Design review of the part shown in the three views and the two pictorial views. Dimensions are in mm from the part's minimum x, y and z. A direction names the side the tool comes from. Coordinates: 2 decimals unless noted, no trailing zeros. Loops run counter-clockwise (first coordinate to the right, second up) from the corner with the lowest first, then second, coordinate; pieces in that order, holes last. Notation, with made-up numbers: M 19.25,82 L 61.25,82 A34 cw 61.25,121 Z; hole C 30,76 d2. An arc over 180 degrees is marked long. Put each result on its own line as item: value. Start each with the question number.
(1) Take a section at D-D, the plane z = 43.5. Give the boundary of the cut face in (x, y), then the cut area to 3 significant figures.
(2) Take a section at A-A, the plane y = 6.35. Give the boundary of the cut face in (x, z) (3 decimals), then the cut area to 3 significant figures.
(3) Clearance check with flat-ended pins moving along their axes: pin 1 (1 mm diameter, centred on x = 5, y = 2, fed in from -Z); pin 2 (1.5 mm diameter, centred on x = 5, z = 12, fed in from -Y); pin 3 (4 mm diameter, centred on x = 5.5, y = 9.5, fed in from -Z); pin 4 (1 mm diameter, centred on y = 3, z = 27.5, fed in from +X). State where each tip first meets the part, or that it passes through.
(4) For probe 1 along Z at (x, y) = (7, 1.5); probe 2 along Y at (x, z) = (6.5, 34.5), list the stretches that pass through material, from the lowest coordinate up. Write a range as [from, to].
(5) For the marked faces 1, 2 and 3, list the 3-axis set-ups (+Z, -Z, +X, -X, +Y, -Y) from which the entire face can be reached by the end or side of a thin tool; tool diameter is ignored.
(6) Take a section at C-C, the plane z = 10.5. Give the boundary of the cut face in (x, y) (3 decimals), then the cut area to 3 significant figures.
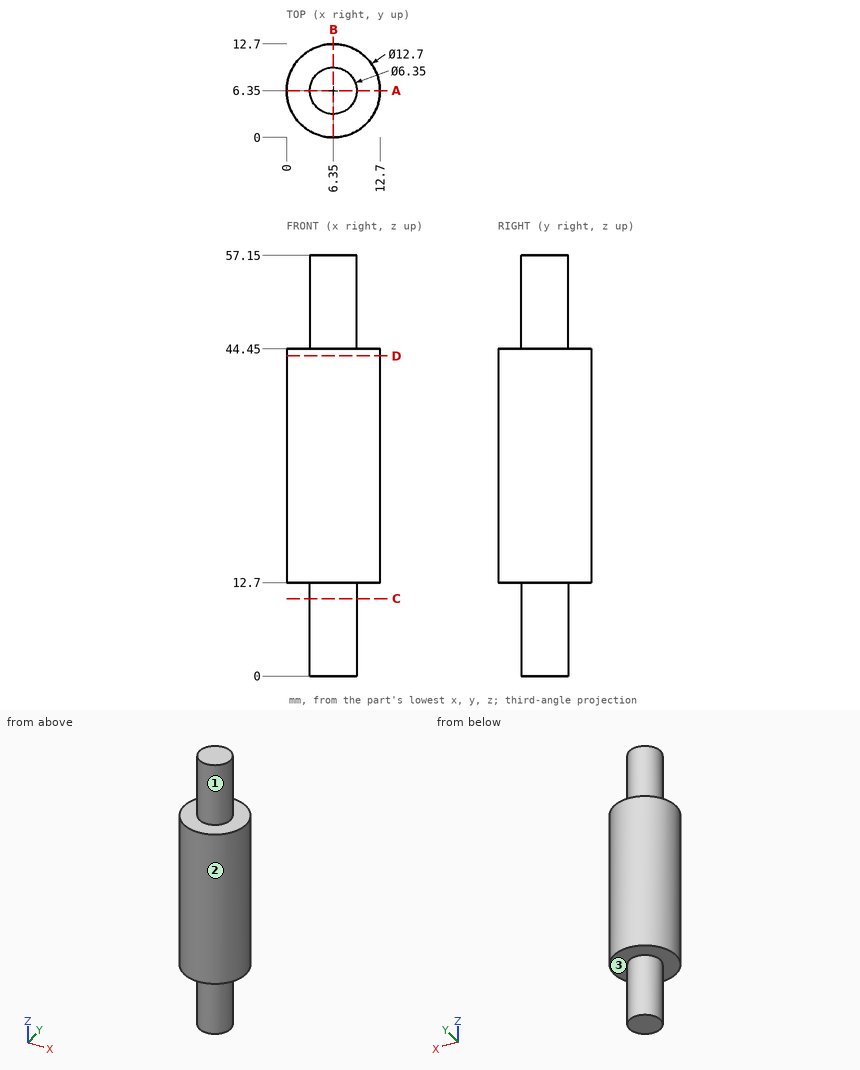
Computed values:
1. outline: C 6.35,6.35 d12.7
1. area: 127 mm^2
2. outline: M 0,12.7 L 3.175,12.7 L 3.175,0 L 9.525,0 L 9.525,12.7 L 12.7,12.7 L 12.7,44.45 L 9.525,44.45 L 9.525,57.15 L 3.175,57.15 L 3.175,44.45 L 0,44.45 Z
2. area: 565 mm^2
3. pin 1: stops at z = 12.7
3. pin 2: stops at y = 0.09
3. pin 3: stops at z = 0
3. pin 4: stops at x = 12.02
4. probe 1: z = [12.7, 44.45]
4. probe 2: y = [0, 12.7]
5. face 1: +Z
5. face 2: +Z, -Z
5. face 3: -Z
6. outline: C 6.35,6.35 d6.35
6. area: 31.7 mm^2
